Source: three-view drawing plus pictorial views. Frame: mm from the lowest corner of the part. A direction names the side the tool comes from. Round coordinates to 2 decimals unless told otherwise and drop trailing zeros. Loops run counter-clockwise (first coordinate to the right, second up) from the corner with the lowest first, then second, coordinate; pieces in that order, holes last. Notation, with made-up numbers: M -2,-35 L 45,-35 A24 cw 45,2 Z; hole C 25,9 d5. An arc over 180 degrees is marked long. Return JSON: item names as keys, results as strings. Group by question number.
1) Section C-C (x = 4). Output: boundary loops of the cut face in (y, z), plus the area to 3 significant figures.
2) Mould query, pull axis X, two halves, no side actions, for the marked faces 1, 2, 3 and 4. Classes: +X half, -X half, draft (parallel to the pull), parting line (faces both ways), or undercut.
3) Section B-B (y = 0.4). Output: boundary loops of the cut face in (x, z).
4) Section D-D (y = 3.6). Output: boundary loops of the cut face in (x, z), plus the area to 3 significant figures.
5) Material intervals for line 1 (Z direction, x = 4, y = 2.5); line 2 (Y direction, x = 0.75, z = 3.5); line 3 (Y direction, x = 2.5, z = 5), sorted ascending. Write a range as from..to.
6) Access query for the marked faces 5, 6 and 7. Directions: +Z, -Z, +X, -X, +Y, -Y. A direction counts if a zero-diameter tool reaches every point of the face in a straight line with its end or side. Return the directions, or none.
7) Contact query for flat-ended pins moving along their axis: P1, Ø1.3, axis at x = 4, z = 4, coming from the -Y side; P2, Ø1.8, axis at x = 3.5, z = 4, coming from the -Y side. Output: stop coordinate, or through.
8) Section A-A (z = 4). Output: boundary loops of the cut face in (x, y), plus the area to 3 significant figures.
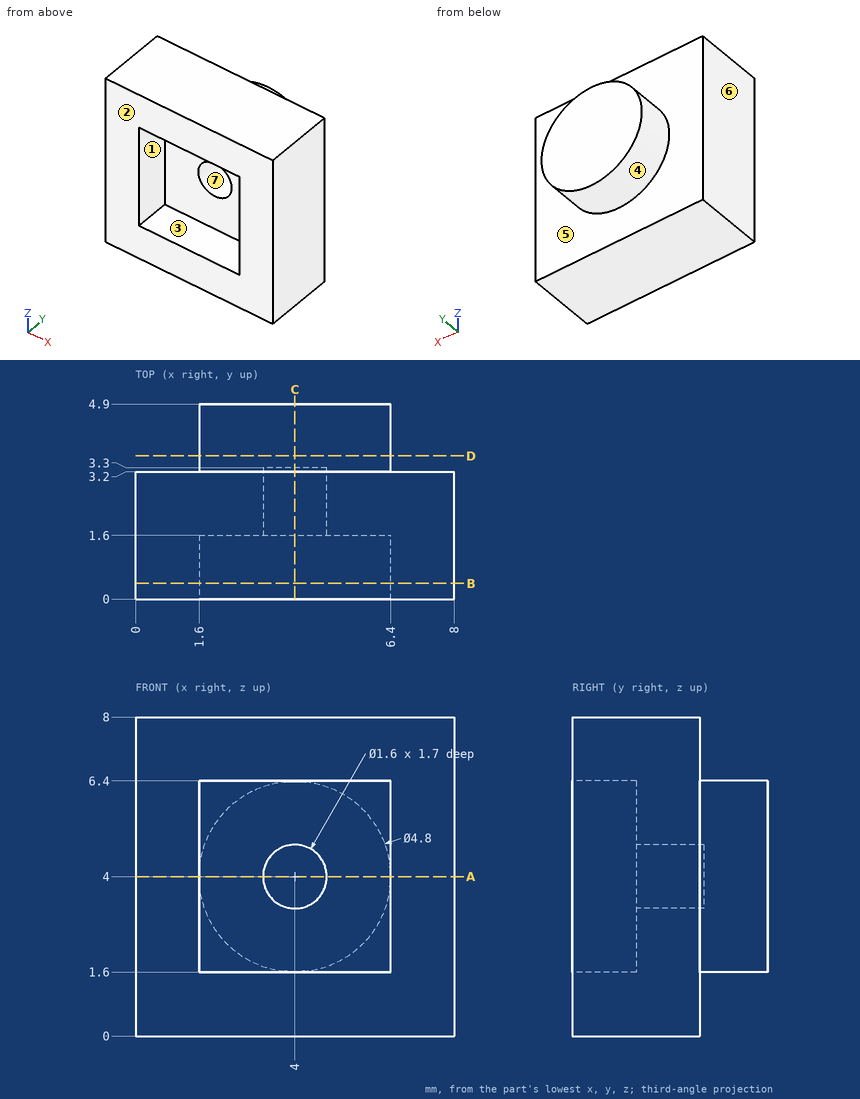
Returned:
{
 "1": {"outline": "M 0,0 L 3.2,0 L 3.2,1.6 L 4.9,1.6 L 4.9,6.4 L 3.2,6.4 L 3.2,8 L 0,8 L 0,6.4 L 1.6,6.4 L 1.6,4.8 L 3.3,4.8 L 3.3,3.2 L 1.6,3.2 L 1.6,1.6 L 0,1.6 Z", "area": "23.4 mm^2"},
 "2": {"face 1": "undercut", "face 2": "draft", "face 3": "undercut", "face 4": "parting line"},
 "3": {"outline": "M 0,0 L 8,0 L 8,8 L 0,8 Z; hole M 1.6,1.6 L 6.4,1.6 L 6.4,6.4 L 1.6,6.4 Z"},
 "4": {"outline": "C 4,4 d4.8", "area": "18.1 mm^2"},
 "5": {"line 1": "z = 0..3.2, 4.8..8", "line 2": "y = 0..3.2", "line 3": "y = 1.6..4.9"},
 "6": {"face 5": "+Y", "face 6": "+Z, -Z, -X, +Y, -Y", "face 7": "-Y"},
 "7": {"P1": "stops at y = 3.3", "P2": "stops at y = 1.6"},
 "8": {"outline": "M 0,0 L 1.6,0 L 1.6,1.6 L 3.2,1.6 L 3.2,3.3 L 4.8,3.3 L 4.8,1.6 L 6.4,1.6 L 6.4,0 L 8,0 L 8,3.2 L 6.4,3.2 L 6.4,4.9 L 1.6,4.9 L 1.6,3.2 L 0,3.2 Z", "area": "23.4 mm^2"}
}
